CAD build for the part. Positions are in the model's coordinates, mm. A direction names the side the tool comes from. Give positions to 0.01 mm unless a question says otherwise; leave off trailing zeros. Order: outer loops, then holes, each group sorted by start corner. A loop starts at its lowest first (then second) coordinate and runs counter-clockwise, first axis right, second up.
Item 1: Two-plate mould, pull along Y, no slides. Class faces 4 (the cylindrical face through (4.652, -5.712, 7.902)), 5 (the flat face through (43, -4, 6)), 6 (the flat face through (42, 0, 0)): released by +Y, released by -Y, zero draft, split by the parting line, or undercut.
Item 2: Flat gauge pins, fed straight in: P1, Ø4, axis at y = -7.5, z = 3.5, coming from the +X side; P2, Ø1, axis at x = 73, z = 9.5, coming from the -Y side; P3, Ø4.5, axis at x = 6.65, y = 5.8, coming from the -Z side. Where does each tip first touch, or does it go through?
Item 3: Band-saw the part on B-B on y = -2. Give the cut face in (x, z).
Item 4: Band-saw the part on A-A on z = 9.5. Give the cut face in (x, y), plus the area to 3 significant figures.
Item 5: Wall check: L1, parallel to Y at x = 78.35, z = 10.5; L2, parallel to X at y = 7, z = 14; L3, parallel to X at y = -6.75, z = 11.25. Give the ranges that are in metal, low to high.
Item 6: Which spindle directions (+Z, -Z, +X, -X, +Y, -Y) get a long thin tool onto all of the face, cutting with end or side? Do faces 1 (the flat face through (9, -10, 8)), 2 (the flat face through (15, 7, 8)), 3 (the cylindrical face through (73.11, -9.69, 7.89)). Say none if no direction does.
Item 7: Band-saw the part on C-C on x = 27.5. Give the cut face in (y, z).
```python
from build123d import *

# Parameters (mm, degrees)
SKETCH_R        = 2
PAD_DEPTH       = 16
CHAMFER_SIZE    = 1
CHAMFER001_SIZE = 1
POCKET_DEPTH    = 16.001
FILLET_R        = 4
FILLET001_R     = 4
FILLET002_R     = 4
FILLET003_R     = 4
FILLET004_R     = 4
SKETCH002_W     = 33
SKETCH002_H     = 10
POCKET001_DEPTH = 3
FILLET005_R     = 1
FILLET006_R     = 1
FILLET007_R     = 1


with BuildPart() as part:
    # Sketch → Pad (new body)
    with BuildSketch(Plane.XY):
        with BuildLine():
            ThreePointArc((7, 10), (2.050253, 7.949747), (0, 3))
            Line((0, -3), (0, 3))
            ThreePointArc((0, -3), (2.050253, -7.949747), (7, -10))
            Line((78, -10), (7, -10))
            ThreePointArc((78, -10), (82.949747, -7.949747), (85, -3))
            Line((85, 3), (85, -3))
            ThreePointArc((85, 3), (82.949747, 7.949747), (78, 10))
            Line((7, 10), (78, 10))
        make_face()
        with Locations((6.65, 5.8)):
            Circle(SKETCH_R, mode=Mode.SUBTRACT)
        with Locations((78.35, 5.8)):
            Circle(SKETCH_R, mode=Mode.SUBTRACT)
        with Locations((6.65, -5.8)):
            Circle(SKETCH_R, mode=Mode.SUBTRACT)
        with Locations((78.35, -5.8)):
            Circle(SKETCH_R, mode=Mode.SUBTRACT)
    extrude(amount=PAD_DEPTH)

    # Chamfer
    chamfer_edges = [part.edges().sort_by_distance(p)[0] for p in [
        (76.35, 5.8, 16),
        (76.35, -5.8, 16),
        (4.65, 5.8, 16),
        (4.65, -5.8, 16),
    ]]
    chamfer(chamfer_edges, length=CHAMFER_SIZE)

    # Chamfer001
    chamfer001_edges = [part.edges().sort_by_distance(p)[0] for p in [
        (4.65, -5.8, 0),
        (76.35, -5.8, 0),
        (76.35, 5.8, 0),
        (4.65, 5.8, 0),
    ]]
    chamfer(chamfer001_edges, length=CHAMFER001_SIZE)

    # Sketch001 (on Face5 of Chamfer001) → Pocket (cut, through all)
    with BuildSketch(Plane.XY.offset(16)):
        Polygon((12, 10), (18, 4), (67, 4), (73, 10), align=None)
        Polygon((12, -10), (73, -10), (67, -4), (18, -4), align=None)
    extrude(amount=-POCKET_DEPTH, mode=Mode.SUBTRACT)

    # Fillet
    fillet_edges = [part.edges().sort_by_distance(p)[0] for p in [
        (12, -10, 8),
    ]]
    fillet(fillet_edges, radius=FILLET_R)

    # Fillet001
    fillet001_edges = [part.edges().sort_by_distance(p)[0] for p in [
        (18, -4, 8),
    ]]
    fillet(fillet001_edges, radius=FILLET001_R)

    # Fillet002
    fillet002_edges = [part.edges().sort_by_distance(p)[0] for p in [
        (73, -10, 8),
        (67, -4, 8),
    ]]
    fillet(fillet002_edges, radius=FILLET002_R)

    # Fillet003
    fillet003_edges = [part.edges().sort_by_distance(p)[0] for p in [
        (12, 10, 8),
        (18, 4, 8),
    ]]
    fillet(fillet003_edges, radius=FILLET003_R)

    # Fillet004
    fillet004_edges = [part.edges().sort_by_distance(p)[0] for p in [
        (73, 10, 8),
        (67, 4, 8),
    ]]
    fillet(fillet004_edges, radius=FILLET004_R)

    # Sketch002 (on Face30 of Fillet004) → Pocket001 (cut)
    with BuildSketch(Plane.XY.offset(16)):
        with Locations((46.5, 0)):
            Rectangle(SKETCH002_W, SKETCH002_H)
    extrude(amount=-POCKET001_DEPTH, mode=Mode.SUBTRACT)

    # Fillet005
    fillet005_edges = [part.edges().sort_by_distance(p)[0] for p in [
        (30, 0, 16),
        (63, 0, 16),
    ]]
    fillet(fillet005_edges, radius=FILLET005_R)

    # Fillet006
    fillet006_edges = [part.edges().sort_by_distance(p)[0] for p in [
        (63, 0, 13),
    ]]
    fillet(fillet006_edges, radius=FILLET006_R)

    # Fillet007
    fillet007_edges = [part.edges().sort_by_distance(p)[0] for p in [
        (30, 0, 13),
    ]]
    fillet(fillet007_edges, radius=FILLET007_R)


solid = part.part
```
The answers:
1. face 4: undercut
1. face 5: released by -Y
1. face 6: zero draft
2. P1: stops at x = 84.54
2. P2: stops at y = -9.83
2. P3: stops at z = 0.75
3. outline: (0, 0) - (85, 0) - (85, 16) - (64, 16) arc R1 ccw to (63, 15) - (63, 14) arc R1 cw to (62, 13) - (31, 13) arc R1 cw to (30, 14) - (30, 15) arc R1 ccw to (29, 16) - (0, 16) - close
4. outline: (0, -3) arc R7 ccw to (7, -10) - (10.34, -10) arc R4 ccw to (13.17, -8.83) - (16.83, -5.17) arc R4 cw to (19.66, -4) - (65.34, -4) arc R4 cw to (68.17, -5.17) - (71.83, -8.83) arc R4 ccw to (74.66, -10) - (78, -10) arc R7 ccw to (85, -3) - (85, 3) arc R7 ccw to (78, 10) - (74.66, 10) arc R4 ccw to (71.83, 8.83) - (68.17, 5.17) arc R4 cw to (65.34, 4) - (19.66, 4) arc R4 cw to (16.83, 5.17) - (13.17, 8.83) arc R4 ccw to (10.34, 10) - (7, 10) arc R7 ccw to (0, 3) - close; hole circle Ø4 at (6.65, -5.8); hole circle Ø4 at (6.65, 5.8); hole circle Ø4 at (78.35, -5.8); hole circle Ø4 at (78.35, 5.8)
4. area: 948 mm2
5. L1: y = -9.99 to -7.8, -3.8 to 3.8, 7.8 to 9.99
5. L2: x = 1.26 to 5.05, 8.25 to 15, 70 to 76.75, 79.95 to 83.74
5. L3: x = 1.09 to 4.89, 8.41 to 15.25, 69.75 to 76.59, 80.11 to 83.91
6. face 1: +Z, -Z, +X, -X, -Y
6. face 2: +Z, -Z, +Y
6. face 3: +Z, -Z, -Y
7. outline: (-4, 0) - (4, 0) - (4, 16) - (-4, 16) - close
